Input: part model. Units: mm. Frame: model coordinates. A direction names the side the tool comes from. Round coordinates to 2 decimals unless told otherwise and drop trailing zeros. Loops run counter-clockwise (first coordinate to the right, second up) from the corner with the lowest first, then second, coordinate; pieces in that order, holes last. Notation, with made-up numbers: (45, 8) -> (60, 8) arc R22 cw to (60, 35) -> close; hole circle Ø9 at (42.25, 61.25). An arc over 180 degrees is marked (long way). Answer as a JSON object with one key per item and string values. Group by question number.
Item 1: Section query A-A on y = 78. Return loops of the section in (x, z).
Item 2: Section query C-C on x = 240. Return loops of the section in (y, z).
Item 3: Section query D-D on x = 62. Return loops of the section in (y, z).
Item 4: Set-up query: faces 1 (the flat face through (-5, 99, 150)), 2 (the flat face through (-340, 106, 2)), 3 (the cylindrical face through (38.698, 100.085, 1.96)). Return all of +Z, -Z, +X, -X, +Y, -Y with unobstructed straight access to the full face (end or side cutting, diameter ignored); none if empty.
Item 5: Pin query (flat end, axial travel): pin 1 (6 mm diameter, centred on y = 175, z = 125, fed in from -X); pin 2 (16 mm diameter, centred on y = 175, z = 125, fed in from +X); pin 3 (8 mm diameter, centred on x = -81.5, z = 24, fed in from +Y). Return the tip coordinate at first contact, or that it passes through.
Item 6: Draft query along X for faces 4 (the flat face through (350, 99, 2)), 5 (the flat face through (-5, 106, 140)), 6 (the flat face through (-2, 200, -145)). Return one class per face: released by +X, released by -X, zero draft, split by the parting line, or undercut.
Item 7: Section query B-B on z = -51. Return loops of the section in (x, y), and give its area (3 significant figures).
Item 8: Material intervals for line 1 (X direction, y = 125.5, z = -4); line 2 (Z direction, x = 11, y = 72); line 3 (Y direction, x = -347, z = 125), sorted ascending. Write a range as [from, to].
from build123d import *

# Parameters (mm, degrees)
CROQUIS1_W              = 700
CROQUIS1_H              = 300
SALIENTE_EXTRUIR1_DEPTH = 200
CROQUIS2_W              = 680
CROQUIS2_H              = 280
CORTAR_EXTRUIR1_DEPTH   = 190
CROQUIS3_R              = 5
CORTAR_EXTRUIR2_DEPTH   = 700
CROQUIS4_R              = 10
SALIENTE_EXTRUIR2_DEPTH = 280


with BuildPart() as part:
    # Croquis1 → Saliente-Extruir1 (new body)
    with BuildSketch(Plane(origin=(0, 0, 0), x_dir=(1, 0, 0), z_dir=(0, 1, 0))):
        Rectangle(CROQUIS1_W, CROQUIS1_H)
    extrude(amount=SALIENTE_EXTRUIR1_DEPTH)

    # Croquis2 → Cortar-Extruir1 (cut)
    with BuildSketch(Plane(origin=(0, 200, 0), x_dir=(1, 0, 0), z_dir=(0, 1, 0))):
        Rectangle(CROQUIS2_W, CROQUIS2_H)
    extrude(amount=-CORTAR_EXTRUIR1_DEPTH, mode=Mode.SUBTRACT)

    # Croquis3 → Cortar-Extruir2 (cut)
    with BuildSketch(Plane(origin=(350, 0, 0), x_dir=(0, 0, -1), z_dir=(1, 0, 0))):
        with Locations((-125, 175)):
            Circle(CROQUIS3_R)
    extrude(amount=-CORTAR_EXTRUIR2_DEPTH, mode=Mode.SUBTRACT)

    # Croquis4 → Saliente-Extruir2 (add)
    with BuildSketch(Plane(origin=(0, 0, 140), x_dir=(-1, 0, 0), z_dir=(0, 0, -1))):
        with Locations(Location((-240, 110, 0), (0, 0, 180))):
            Circle(CROQUIS4_R)
        with Locations(Location((-140, 110, 0), (0, 0, 180))):
            Circle(CROQUIS4_R)
        with Locations(Location((-40, 110, 0), (0, 0, 180))):
            Circle(CROQUIS4_R)
        with Locations(Location((140, 110, 0), (0, 0, 180))):
            Circle(CROQUIS4_R)
        with Locations(Location((240, 110, 0), (0, 0, 180))):
            Circle(CROQUIS4_R)
        with Locations(Location((40, 110, 0), (0, 0, 180))):
            Circle(CROQUIS4_R)
    extrude(amount=SALIENTE_EXTRUIR2_DEPTH)


solid = part.part
Solved:
{
 "1": {"outline": "(-350, -150) -> (350, -150) -> (350, 150) -> (-350, 150) -> close; hole (-340, -140) -> (340, -140) -> (340, 140) -> (-340, 140) -> close"},
 "2": {"outline": "(0, -150) -> (200, -150) -> (200, -140) -> (120, -140) -> (120, 140) -> (200, 140) -> (200, 150) -> (0, 150) -> close; hole (10, -140) -> (100, -140) -> (100, 140) -> (10, 140) -> close"},
 "3": {"outline": "(0, -150) -> (200, -150) -> (200, -140) -> (10, -140) -> (10, 140) -> (200, 140) -> (200, 150) -> (0, 150) -> close"},
 "4": {"face 1": "+Z, +X, -X, +Y, -Y", "face 2": "+Y", "face 3": "none"},
 "5": {"pin 1": "through", "pin 2": "x = 350", "pin 3": "y = 10"},
 "6": {"face 4": "released by +X", "face 5": "undercut", "face 6": "zero draft"},
 "7": {"outline": "(-350, 0) -> (350, 0) -> (350, 200) -> (340, 200) -> (340, 10) -> (-340, 10) -> (-340, 200) -> (-350, 200) -> close; circle Ø20 at (-240, 110); circle Ø20 at (-140, 110); circle Ø20 at (-40, 110); circle Ø20 at (40, 110); circle Ø20 at (140, 110); circle Ø20 at (240, 110)", "area": "12,700 mm²"},
 "8": {"line 1": "[-350, -340], [340, 350]", "line 2": "[-150, -140], [140, 150]", "line 3": "[0, 170], [180, 200]"}
}
